Design review of the part built by this model. Coordinates are the model's own, in mm. A direction names the side the tool comes from. Round coordinates to 2 decimals unless told otherwise and drop trailing zeros. Loops run counter-clockwise (first coordinate to the right, second up) from the corner with the lowest first, then second, coordinate; pieces in that order, holes last. Notation, with made-up numbers: (48.5, 80.5) -> (64.5, 80.5) arc R25 ccw to (64.5, 95.5) -> close; hole circle Ø9 at (84.5, -1). An arc over 180 degrees is marked (long way). Answer as CSV lines item,"result". Start each with the question number.
(1) Take a section at A-A, the plane y = 1.3. Write out the cut boundary in (x, z), and give its area (3 significant figures).
(2) Take a section at C-C, the plane x = 5. Write out the cut boundary in (y, z).
(3) For P1, Ø1.2, axis at x = 58, y = 2, coming from the -Z side; P2, Ø1.2, axis at x = -58, y = 1, coming from the +Z side; P3, Ø1.5, axis at y = 0.5, z = 2.5, coming from the -X side, all flat-tipped, find the tip position at first contact; note any pin that passes through.
(4) To check wall thickness, follow line 1 (X direction, y = 1.25, z = 21.5); line 2 (Z direction, x = -29, y = 0.7); line 3 (X direction, y = 2.4, z = 18.75). State the ranges of each line that lie inside material, in increasing order. Write a range as from..to.
(5) Take a section at B-B, the plane z = 4. Write out the cut boundary in (x, y), and give its area (4 significant figures).
(6) Machinability: for faces 1 (the face through (56.25, 1, 3)), 2 (the face through (48.25, 1, 22)), 3 (the face through (57, 1, 15.25)), 4 (the face through (-56.25, 1, 3)), 5 (the face through (-54, 1, 21)), which of the approach directions +Z, -Z, +X, -X, +Y, -Y give a long, thin tool a straight path to every point of the face, cutting with its end or side? Answer none if there is none.
from build123d import *

# Parameters (mm, degrees)
SKETCH_1_W      = 3
SKETCH_1_H      = 3
EXTRUDE_1_DEPTH = 3
FILLET_1_R      = 0.5


with BuildPart() as part:
    # Эскиз1 → Бобышка-Вытянуть1 (new body)
    with BuildSketch(Plane(origin=(0, 0, 0), x_dir=(1, 0, 0), z_dir=(0, 1, 0))):
        Polygon((-56.25, -21), (56.25, -21), (56.25, -15.25), (59.25, -15.25), (59.25, -5.25), (56.25, -5.25), (56.25, 0), (-56.25, 0), (-56.25, -5.25), (-59.25, -5.25), (-59.25, -15.25), (-56.25, -15.25), align=None)
        with Locations((49.75, -22.5)):
            Rectangle(SKETCH_1_W, SKETCH_1_H)
        with Locations((-49.75, -22.5)):
            Rectangle(SKETCH_1_W, SKETCH_1_H)
    extrude(amount=EXTRUDE_1_DEPTH)

    # Скругление1
    fillet_1_edges = [part.edges().sort_by_distance(p)[0] for p in [
        (-59.25, 1.5, 15.25),
        (-59.25, 1.5, 5.25),
        (59.25, 1.5, 5.25),
        (59.25, 1.5, 15.25),
        (51.25, 1.5, 24),
        (48.25, 1.5, 24),
        (-48.25, 1.5, 24),
        (-51.25, 1.5, 24),
    ]]
    fillet(fillet_1_edges, radius=FILLET_1_R)


solid = part.part
The answers:
1,outline,"(-59.25, 5.75) arc R0.5 ccw to (-58.75, 5.25) -> (-56.25, 5.25) -> (-56.25, 0) -> (56.25, 0) -> (56.25, 5.25) -> (58.75, 5.25) arc R0.5 ccw to (59.25, 5.75) -> (59.25, 14.75) arc R0.5 ccw to (58.75, 15.25) -> (56.25, 15.25) -> (56.25, 21) -> (51.25, 21) -> (51.25, 23.5) arc R0.5 ccw to (50.75, 24) -> (48.75, 24) arc R0.5 ccw to (48.25, 23.5) -> (48.25, 21) -> (-48.25, 21) -> (-48.25, 23.5) arc R0.5 ccw to (-48.75, 24) -> (-50.75, 24) arc R0.5 ccw to (-51.25, 23.5) -> (-51.25, 21) -> (-56.25, 21) -> (-56.25, 15.25) -> (-58.75, 15.25) arc R0.5 ccw to (-59.25, 14.75) -> close"
1,area,"2,440 mm²"
2,outline,"(0, 0) -> (3, 0) -> (3, 21) -> (0, 21) -> close"
3,P1,"z = 5.25"
3,P2,"z = 15.25"
3,P3,"x = -56.25"
4,line 1,"-51.25..-48.25, 48.25..51.25"
4,line 2,"0..21"
4,line 3,"-56.25..56.25"
5,outline,"(-56.25, 0) -> (56.25, 0) -> (56.25, 3) -> (-56.25, 3) -> close"
5,area,"337.5 mm²"
6,face 1,"-Z, +X, +Y, -Y"
6,face 2,"+Z, +Y, -Y"
6,face 3,"+Z, +X, +Y, -Y"
6,face 4,"-Z, -X, +Y, -Y"
6,face 5,"+Z, -X, +Y, -Y"
